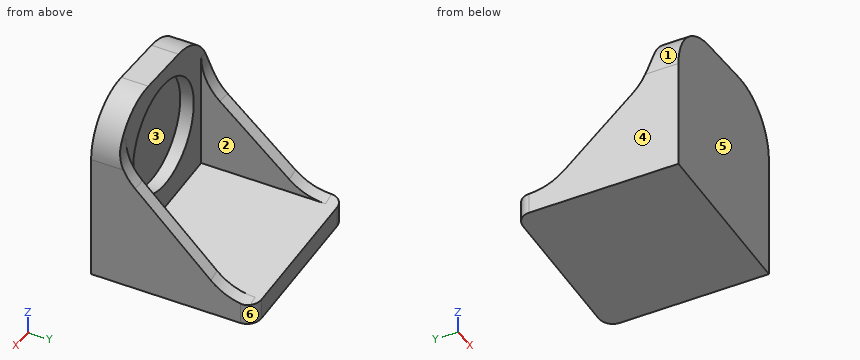
from build123d import *

# Parameters (mm, degrees)
BOSS_EXTRUDE1_DEPTH = 6.35
SKETCH2_R           = 12.7635
CUT_EXTRUDE1_DEPTH  = 3.175
BOSS_EXTRUDE2_DEPTH = 31.75
FILLET1_R           = 12.7
BOSS_EXTRUDE3_DEPTH = 3.175
BOSS_EXTRUDE7_DEPTH = 3.175
FILLET2_R           = 12.7
FILLET3_R           = 3.175


with BuildPart() as part:
    # Sketch1 → Boss-Extrude1 (new body)
    with BuildSketch(Plane(origin=(0, 0, 0), x_dir=(1, 0, 0), z_dir=(0, 1, 0))):
        Polygon((-19.05, 19.05), (-19.05, -19.05), (19.05, -19.05), (19.05, 22.651510368), align=None)
    extrude(amount=BOSS_EXTRUDE1_DEPTH)

    # Sketch2 → Cut-Extrude1 (cut)
    with BuildSketch(Plane(origin=(0, 6.35, 0), x_dir=(1, 0, 0), z_dir=(0, 1, 0))):
        with Locations(Location((0, -2.54, 0), (0, 0, 270))):
            Circle(SKETCH2_R)
    extrude(amount=-CUT_EXTRUDE1_DEPTH, mode=Mode.SUBTRACT)

    # Sketch3 → Boss-Extrude2 (add)
    with BuildSketch(Plane(origin=(0, 6.35, 0), x_dir=(1, 0, 0), z_dir=(0, 1, 0))):
        Polygon((19.05, 22.651510368), (-19.05, 19.05), (-19.05, 14.2875), (19.05, 17.889010368), align=None)
    extrude(amount=BOSS_EXTRUDE2_DEPTH)

    # Fillet1
    fillet1_edges = [part.edges().sort_by_distance(p)[0] for p in [
        (19.05, 3.175, 19.05),
        (-19.05, 3.175, 19.05),
    ]]
    fillet(fillet1_edges, radius=FILLET1_R)

    # Sketch4 → Boss-Extrude3 (add)
    with BuildSketch(Plane(origin=(19.05, 0, 0), x_dir=(0, 0, -1), z_dir=(1, 0, 0))):
        Polygon((-6.35, 6.35), (17.889010368, 31.75), (17.889010368, 6.35), align=None)
    extrude(amount=-BOSS_EXTRUDE3_DEPTH)

    # Sketch6 → Boss-Extrude7 (add)
    with BuildSketch(Plane.ZY.offset(19.05)):
        Polygon((-15.5575, 31.75), (6.35, 6.35), (-15.5575, 6.35), align=None)
    extrude(amount=-BOSS_EXTRUDE7_DEPTH)

    # Fillet2
    fillet2_edges = [part.edges().sort_by_distance(p)[0] for p in [
        (17.4625, 6.35, 6.35),
        (17.4625, 31.592749419, -17.738947436),
        (-17.4625, 6.35, 6.35),
        (-17.4625, 30.45152224, -14.437562932),
    ]]
    fillet(fillet2_edges, radius=FILLET2_R)

    # Fillet3
    fillet3_edges = [part.edges().sort_by_distance(p)[0] for p in [
        (19.05, 38.1, -20.270260368),
        (-19.05, 38.1, -16.66875),
    ]]
    fillet(fillet3_edges, radius=FILLET3_R)


solid = part.part
CAD build for the part. Positions are in the model's coordinates, mm. Face numbers are marked on the shaded views. A direction names the side the tool comes from. Round coordinates to 2 decimals unless told otherwise and drop trailing zeros. Loops run counter-clockwise (first coordinate to the right, second up) from the corner with the lowest first, then second, coordinate; pieces in that order, holes last. Notation, with made-up numbers: M 36.25,69 L 42.25,69 A11 ccw 42.25,85 Z; hole C 23.25,-14 d3. An arc over 180 degrees is marked long. One line per question, with ' | ' between items. Start each with the question number.
Item 1: Which spindle directions (+Z, -Z, +X, -X, +Y, -Y) get a long thin tool onto all of the face, cutting with end or side? Do the marked faces 1 and 2. Say none if no direction does.
Item 2: Cut at C-C, the plane z = 9.5. Write the cut outline in (x, y) (3 decimals), plus the area to 3 significant figures.
Item 3: Cut at A-A, the plane x = -2.5. Write the cut outline in (y, z) (3 decimals).
Item 4: Two-plate mould, pull along X, no slides. Class the marked faces 3, 4, 5 and 6: pulls with the +X half, pulls with the -X half, needs draft (parallel to the pull), parting line crosses it, or undercut.
Item 5: Cut at B-B, the plane y = 13. Write the cut outline in (x, z) (3 decimals).
Item 6: Wall check: line 1 (X direction, y = 10, z = -13) (3 decimals); line 2 (X direction, y = 5, z = 2); line 3 (Y direction, x = 6, z = 7) (3 decimals). Give the ranges that are in metal, low to high.
Item 7: Pin check, flat tips, straight feed: pin 1 Ø5 at (x, z) = (-7, -0.5) entering from +Y (3 decimals); pin 2 Ø1.5 at (x, y) = (-4, 24.5) entering from -Z; pin 3 Ø6 at (x, y) = (5.5, 12) entering from +Z. Stop position of each tip, or through.
Responses:
1) face 1: +Z, -X, +Y, -Y | face 2: +Z, +Y
2) outline: M -18.653,0 L 18.653,0 L 18.653,6.557 L 15.875,6.557 L 15.875,6.35 L 10.699,6.35 L 10.699,3.175 L -10.699,3.175 L -10.699,6.35 L -15.875,6.35 L -15.875,6.633 L -18.653,6.633 Z | area: 170 mm²
3) outline: M 0,-20.614 L 38.1,-20.614 L 38.1,-15.852 L 6.35,-15.852 L 6.35,-9.976 L 3.175,-9.976 L 3.175,15.056 L 6.35,15.056 L 6.35,19.05 L 0,19.05 Z
4) face 3: undercut | face 4: pulls with the -X half | face 5: needs draft | face 6: pulls with the +X half
5) outline: M -19.05,-19.05 L 19.05,-22.652 L 19.05,0.004 L 15.875,0.004 L 15.875,-17.589 L -15.875,-14.588 L -15.875,0.614 L -19.05,0.614 Z
6) line 1: x = -19.05 to -15.875, 15.875 to 19.05 | line 2: x = -19.05 to -12.75, 12.75 to 19.05 | line 3: y = 0 to 3.175
7) pin 1: stops at y = 3.175 | pin 2: stops at z = -20.54 | pin 3: stops at z = -16.32
